Read the model definition and answer for the solid it produces. Units are mm, in the model's axes. A direction names the side the tool comes from. Coordinates: 2 decimals unless noted, no trailing zeros. Write each loop counter-clockwise with the first axis right and the second up, starting at its lowest first coordinate (ties: lowest second). Pieces come first, ordered by that corner, then holes. Notation, with made-up numbers: (-31.75, 77.25) -> (-19.75, 77.25) arc R32 cw to (-19.75, 106.25) -> close; hole circle Ø6 at (16, 58.5). An arc over 180 degrees is marked (long way). One line per item, written item: value. Start each with the question number.
1. For a pull along X with two mould halves and no side action, classify faces 5 (the flat face through (6, -4, 29)), 6 (the flat face through (5, -5, -1)), 7 (the flat face through (10, -5, 20.5)), 8 (the flat face through (-1, -10, 16)) as pulls with the +X half, pulls with the -X half, needs draft (parallel to the pull), parting line crosses it, or undercut.
2. Find section A-A, the plane y = -4.5. Write down the section's boundary in (x, z), and give its area (3 significant figures).
3. Given P1, Ø1.5, axis at x = 12.5, y = -1, coming from the -Z side; P2, Ø6, axis at y = -2.5, z = 11.5, coming from the +X side; P3, Ø2.5, axis at x = 3.5, y = -4, coming from the +Z side, each flat-ended and moving along its own axis, determine where each tip first touches the part or whether it passes through.
4. For faces 1 (the flat face through (-2, -7, 26)), 2 (the flat face through (20.5, -5, 20)), 3 (the flat face through (0, -6, 29)), 4 (the flat face through (9, -4, 29)), determine the directions among +Z, -Z, +X, -X, +Y, -Y from which every point of the face is accessible in a straight line to the end or side of a thin tool.
5. Find section B-B, the plane y = -7.5. Write down the section's boundary in (x, z).
6. Find section D-D, the plane x = 17.5. Write down the section's boundary in (y, z).
7. Consider line 1 along X through (y, z) = (-6.25, 29); line 2 along Z through (x, y) = (4, -6.5); line 3 along Z through (x, y) = (-0.25, -2.5). Determine where each line is inside the solid, lowest interval first.
8. Find section C-C, the plane z = 3. Write down the section's boundary in (x, y), and give its area (3 significant figures).
```python
from build123d import *

# Parameters (mm, degrees)
F1_DEPTH = 10
F2_R     = 1
F3_W     = 7
F3_H     = 5
F4_DEPTH = 3
F5_W     = 7
F5_H     = 5
F6_DEPTH = 3


with BuildPart() as f1:
    # F0 (on Front) → F1 (new body)
    with BuildSketch(Plane.XZ):
        Polygon((5, -3), (5, 0), (0, 0), (0, 20.5), (20.5, 20.5), (20.5, 18.5), (23.5, 20.5), (23.5, 23.5), (9, 23.5), (9, 30.5), (6, 30.5), (6, 23.5), (0, 23.5), (0, 30.5), (-3, 30.5), (-3, 23.5), (-3, -3), align=None)
    extrude(amount=F1_DEPTH)

    # F2
    f2_edges = [f1.edges().sort_by_distance(p)[0] for p in [
        (23.5, -5, 23.5),
        (-3, -5, -3),
        (23.5, -5, 20.5),
        (5, -5, -3),
    ]]
    fillet(f2_edges, radius=F2_R)

    # F3 (on face) → F4 (cut, through all)
    with BuildSketch(Plane(origin=(-3, 0, 0), x_dir=(0, -1, 0), z_dir=(-1, 0, 0))):
        with Locations((3.5, 26)):
            Rectangle(F3_W, F3_H)
    extrude(amount=-F4_DEPTH, mode=Mode.SUBTRACT)

    # F5 (on face) → F6 (cut, through all)
    with BuildSketch(Plane.YZ.offset(9)):
        with Locations((-6.5, 26)):
            Rectangle(F5_W, F5_H)
    extrude(amount=-F6_DEPTH, mode=Mode.SUBTRACT)


solid = f1.part
```
Answer block:
1. face 5: undercut
1. face 6: pulls with the +X half
1. face 7: undercut
1. face 8: needs draft
2. outline: (-3, -2) arc R1 ccw to (-2, -3) -> (4, -3) arc R1 ccw to (5, -2) -> (5, 0) -> (0, 0) -> (0, 20.5) -> (20.5, 20.5) -> (20.5, 18.5) -> (23.05, 20.2) arc R1 ccw to (23.5, 21.04) -> (23.5, 22.5) arc R1 ccw to (22.5, 23.5) -> (-3, 23.5) -> close; (-3, 28.5) -> (0, 28.5) -> (0, 30.5) -> (-3, 30.5) -> close; (6, 28.5) -> (9, 28.5) -> (9, 30.5) -> (6, 30.5) -> close
2. area: 179 mm2
3. P1: stops at z = 20.5
3. P2: stops at x = 0
3. P3: stops at z = 23.5
4. face 1: +X, -X, +Y
4. face 2: -Z, +Y, -Y
4. face 3: +Z, +Y, -Y
4. face 4: +Z, +X, +Y, -Y
5. outline: (-3, -2) arc R1 ccw to (-2, -3) -> (4, -3) arc R1 ccw to (5, -2) -> (5, 0) -> (0, 0) -> (0, 20.5) -> (20.5, 20.5) -> (20.5, 18.5) -> (23.05, 20.2) arc R1 ccw to (23.5, 21.04) -> (23.5, 22.5) arc R1 ccw to (22.5, 23.5) -> (0, 23.5) -> (0, 30.5) -> (-3, 30.5) -> close; (6, 28.5) -> (9, 28.5) -> (9, 30.5) -> (6, 30.5) -> close
6. outline: (-10, 20.5) -> (0, 20.5) -> (0, 23.5) -> (-10, 23.5) -> close
7. line 1: x = -3 to 0, 6 to 9
7. line 2: z = -3 to 0, 20.5 to 23.5
7. line 3: z = -3 to 23.5, 28.5 to 30.5
8. outline: (-3, -10) -> (0, -10) -> (0, 0) -> (-3, 0) -> close
8. area: 30.0 mm2
